Can you work these out from the model? Positions are in its coordinate system, mm. A direction names the side the tool comes from. Round coordinates to 2 decimals unless told otherwise and drop trailing zeros. Loops run counter-clockwise (first coordinate to the right, second up) from the corner with the lowest first, then second, coordinate; pieces in that order, holes last. Notation, with made-up numbers: (-25.5, 56.25) -> (-14.5, 56.25) arc R19 ccw to (-14.5, 83.25) -> close; hole circle Ø1 at (-7.5, -19.75). An arc over 180 degrees is marked (long way). Write item = value, one per line.
from build123d import *

# Parameters (mm, degrees)
F0_W     = 100
F0_H     = 100
F1_DEPTH = 25
F2_R     = 3
F3_DEPTH = 7
F4_R     = 1.75
F5_DEPTH = 25


with BuildPart() as f1:
    # F0 (on Top) → F1 (new body)
    with BuildSketch(Plane.XY):
        Rectangle(F0_W, F0_H)
    extrude(amount=F1_DEPTH)

    # F2 (on face) → F3 (cut)
    with BuildSketch(Plane.XY.offset(25)):
        Circle(F2_R)
    extrude(amount=-F3_DEPTH, mode=Mode.SUBTRACT)

    # F4 (on face) → F5 (cut)
    with BuildSketch(Plane.XY.offset(18)):
        Circle(F4_R)
    extrude(amount=-F5_DEPTH, mode=Mode.SUBTRACT)

    # F6 (on Right) → F7 (revolve, cut)
    with BuildSketch(Plane.YZ):
        Polygon((0, 18), (0, 25), (-3.5, 25), (-2.265711, 18), align=None)
    revolve(axis=Axis((0, 0, 21.5), (0, 0, 1)), mode=Mode.SUBTRACT)


solid = f1.part
1. For faces 5 (the flat face through (-50, -1, 12)), 6 (the cylindrical face through (-0.65, -2.93, 20.11)), which set-ups out of +Z, -Z, +X, -X, +Y, -Y let a thin tool reach every point of the face, with its end or its side?
Entries:
face_5 = +Z, -Z, -X, +Y, -Y
face_6 = +Z
2. Suppose I cut it at A-A, the plane y = 0. List the corners of the cut face in (x, z) for me, and give its area (3 significant figures).
Entries:
outline = (-50, 0) -> (-1.75, 0) -> (-1.75, 18) -> (-3, 18) -> (-3, 22.16) -> (-3.5, 25) -> (-50, 25) -> close; (1.75, 0) -> (50, 0) -> (50, 25) -> (3.5, 25) -> (3, 22.16) -> (3, 18) -> (1.75, 18) -> close
area = 2,390 mm²
3. We'd pull the mould along Y, two halves only. Please class faces 1 (the flat face through (-1, 50, 12)), 2 (the flat face through (0, -2, 18)), 3 (the flat face through (-1, 12, 0)), 4 (the cylindrical face through (1.617, -0.67, 9.126)): released by +Y, released by -Y, zero draft, split by the parting line, or undercut.
Entries:
face_1 = released by +Y
face_2 = undercut
face_3 = zero draft
face_4 = undercut
4. I need wall thicknesses on line 1 (Y direction, x = 0, z = 20.35); line 2 (Y direction, x = 0, z = 8.75). Which ranges of each line are inside material? Lowest first, please. Write a range as [from, to].
Entries:
line_1 = [-50, -3], [3, 50]
line_2 = [-50, -1.75], [1.75, 50]
